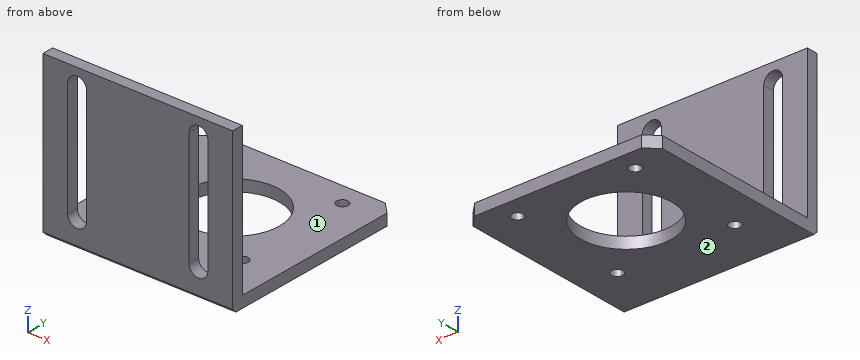
```python
from build123d import *

# Parameters (mm, degrees)
SKETCH1_R           = 12
SKETCH1_R_2         = 1.5
BOSS_EXTRUDE1_DEPTH = 3
BOSS_EXTRUDE2_DEPTH = 3
SKETCH3_W           = 50
SKETCH3_H           = 3
BOSS_EXTRUDE3_DEPTH = 39
CHAMFER1_SIZE       = 1
CUT_EXTRUDE1_DEPTH  = 3


with BuildPart() as part:
    # Sketch1 → Boss-Extrude1 (new body)
    with BuildSketch(Plane.XY):
        Polygon((-22, 21.15), (-25, 18.15), (-25, -23.85), (-22, -26.85), (22, -26.85), (25, -23.85), (25, 18.15), (22, 21.15), align=None)
        Circle(SKETCH1_R, mode=Mode.SUBTRACT)
        with Locations((-15.5, 15.5)):
            Circle(SKETCH1_R_2, mode=Mode.SUBTRACT)
        with Locations((15.5, 15.5)):
            Circle(SKETCH1_R_2, mode=Mode.SUBTRACT)
        with Locations((-15.5, -15.5)):
            Circle(SKETCH1_R_2, mode=Mode.SUBTRACT)
        with Locations((15.5, -15.5)):
            Circle(SKETCH1_R_2, mode=Mode.SUBTRACT)
    extrude(amount=BOSS_EXTRUDE1_DEPTH)

    # Sketch2 → Boss-Extrude2 (add)
    with BuildSketch(Plane(origin=(0, 0, 0), x_dir=(-1, 0, 0), z_dir=(0, 0, -1))):
        Polygon((-25, -23.85), (-25, -29.85), (25, -29.85), (25, -23.85), (22, -26.85), (-22, -26.85), align=None)
    extrude(amount=-BOSS_EXTRUDE2_DEPTH)

    # Sketch3 → Boss-Extrude3 (add)
    with BuildSketch(Plane.XY.offset(3)):
        with Locations((0, -28.35)):
            Rectangle(SKETCH3_W, SKETCH3_H)
    extrude(amount=BOSS_EXTRUDE3_DEPTH)

    # Chamfer1
    chamfer1_edges = [part.edges().sort_by_distance(p)[0] for p in [
        (0, -29.85, 0),
    ]]
    chamfer(chamfer1_edges, length=CHAMFER1_SIZE)

    # Sketch4 → Cut-Extrude1 (cut)
    with BuildSketch(Plane(origin=(0, -26.85, 0), x_dir=(1, 0, 0), z_dir=(0, 1, 0))):
        with BuildLine():
            Line((18.5, -7.5), (18.5, -37.5))
            ThreePointArc((18.5, -37.5), (16, -40), (13.5, -37.5))
            Line((13.5, -37.5), (13.5, -7.5))
            ThreePointArc((13.5, -7.5), (16, -5), (18.5, -7.5))
        make_face()
        with BuildLine():
            Line((-18.5, -7.5), (-18.5, -37.5))
            ThreePointArc((-18.5, -37.5), (-16, -40), (-13.5, -37.5))
            Line((-13.5, -37.5), (-13.5, -7.5))
            ThreePointArc((-13.5, -7.5), (-16, -5), (-18.5, -7.5))
        make_face()
    extrude(amount=-CUT_EXTRUDE1_DEPTH, mode=Mode.SUBTRACT)


solid = part.part
```
Read the model definition and answer for the solid it produces. Units are mm, in the model's axes. Face numbers are marked on the shaded views. A direction names the side the tool comes from. Give positions to 0.01 mm unless a question says otherwise; leave off trailing zeros. Order: outer loops, then holes, each group sorted by start corner. A loop starts at its lowest first (then second) coordinate and runs counter-clockwise, first axis right, second up.
(1) Find section D-D (x = -15.5). Give the vertices of the cut face in (y, z), plus the area to 3 significant figures.
(2) Given pin 1 (4 mm diameter, centred on x = 9.5, y = 11.5, fed in from +Z); pin 2 (1.5 mm diameter, centred on x = 3.5, z = 8.5, fed in from +Y), each flat-ended and moving along its own axis, determine where each tip first touches the part or whether it passes through.
(3) Straight lines are drawn through the part: L1, parallel to X at y = 15, z = 2; L2, parallel to Y at x = -21, z = 5.5; L3, parallel to Y at x = 0, z = 1. For each, find the intervals that lie inside material, in ascending order.
(4) For the marked faces 1 and 2, determine the directions among +Z, -Z, +X, -X, +Y, -Y from which every point of the face is accessible in a straight line to the end or side of a thin tool.
(5) Find section C-C (y = 15.5). Give the vertices of the cut face in (x, z).
(6) Find section B-B (x = 0). Give the vertices of the cut face in (y, z), plus the area to 4 significant figures.
(7) Find section A-A (z = 34). Give the vertices of the cut face in (x, y), plus the area to 3 significant figures.
Result sheet:
1. outline: (-29.85, 1) - (-28.85, 0) - (-17, 0) - (-17, 3) - (-26.85, 3) - (-26.85, 5.05) - (-29.85, 5.05) - close; (-29.85, 39.95) - (-26.85, 39.95) - (-26.85, 42) - (-29.85, 42) - close; (-14, 0) - (14, 0) - (14, 3) - (-14, 3) - close; (17, 0) - (21.15, 0) - (21.15, 3) - (17, 3) - close
1. area: 147 mm2
2. pin 1: stops at z = 3
2. pin 2: stops at y = -26.85
3. L1: x = -25 to -16.91, -14.09 to 14.09, 16.91 to 25
3. L2: y = -29.85 to -26.85
3. L3: y = -29.85 to -12, 12 to 21.15
4. face 1: +Z, +X, -X, +Y
4. face 2: -Z, +X, -X, +Y, -Y
5. outline: (-25, 0) - (-17, 0) - (-17, 3) - (-25, 3) - close; (-14, 0) - (14, 0) - (14, 3) - (-14, 3) - close; (17, 0) - (25, 0) - (25, 3) - (17, 3) - close
6. outline: (-29.85, 1) - (-28.85, 0) - (-12, 0) - (-12, 3) - (-26.85, 3) - (-26.85, 42) - (-29.85, 42) - close; (12, 0) - (21.15, 0) - (21.15, 3) - (12, 3) - close
6. area: 197.5 mm2
7. outline: (-25, -29.85) - (-18.5, -29.85) - (-18.5, -26.85) - (-25, -26.85) - close; (-13.5, -29.85) - (13.5, -29.85) - (13.5, -26.85) - (-13.5, -26.85) - close; (18.5, -29.85) - (25, -29.85) - (25, -26.85) - (18.5, -26.85) - close
7. area: 120 mm2
